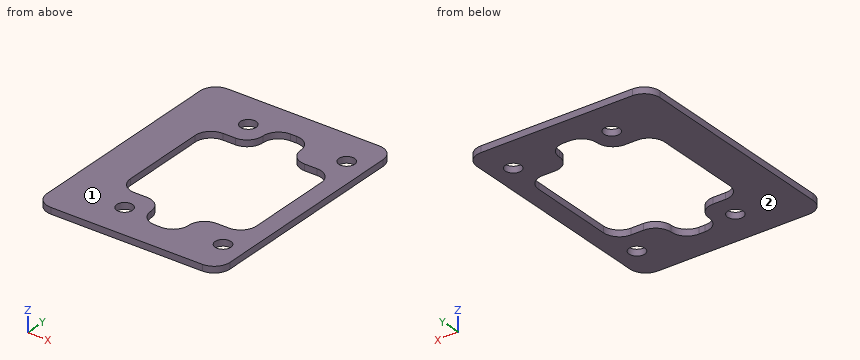
from build123d import *

# Parameters (mm, degrees)
SKETCH1_W       = 23.25
SKETCH1_H       = 30
SKETCH1_R       = 1
BODY_DEPTH      = 0.8
CORNER_FILLET_R = 2
CUTOUT_DEPTH    = 49.678263528
CUTOUT_FILLET_R = 2


with BuildPart() as part:
    # Sketch1 → body (new body)
    with BuildSketch(Plane.XY):
        with Locations((16.812358178, 24.5)):
            Rectangle(SKETCH1_W, SKETCH1_H)
        with Locations((25.687358178, 14)):
            Circle(SKETCH1_R, mode=Mode.SUBTRACT)
        with Locations(Location((25.687358178, 35, 0), (0, 0, 180))):
            Circle(SKETCH1_R, mode=Mode.SUBTRACT)
        with Locations(Location((13.187358178, 14, 0), (0, 0, 180))):
            Circle(SKETCH1_R, mode=Mode.SUBTRACT)
        with Locations((13.187358178, 35)):
            Circle(SKETCH1_R, mode=Mode.SUBTRACT)
    extrude(amount=BODY_DEPTH)

    # corner fillet
    corner_fillet_edges = [part.edges().sort_by_distance(p)[0] for p in [
        (5.187358178, 39.5, 0.4),
        (28.437358178, 39.5, 0.4),
        (28.437358178, 9.5, 0.4),
        (5.187358178, 9.5, 0.4),
    ]]
    fillet(corner_fillet_edges, radius=CORNER_FILLET_R)

    # Sketch2 → cutout (cut, through all)
    with BuildSketch(Plane(origin=(0, 0, 0), x_dir=(-1, 0, 0), z_dir=(0, 0, -1))):
        Polygon((-26.187358178, 17), (-26.187358178, 32), (-20.587358178, 32), (-20.587358178, 36), (-15.787358178, 36), (-15.787358178, 32), (-10.187358178, 32), (-10.187358178, 17), (-15.787358178, 17), (-15.787358178, 13), (-20.587358178, 13), (-20.587358178, 17), align=None)
    extrude(amount=-CUTOUT_DEPTH, mode=Mode.SUBTRACT)

    # cutout fillet
    cutout_fillet_edges = [part.edges().sort_by_distance(p)[0] for p in [
        (26.187358178, 32, 0.4),
        (20.587358178, 32, 0.4),
        (20.587358178, 36, 0.4),
        (15.787358178, 36, 0.4),
        (15.787358178, 32, 0.4),
        (10.187358178, 32, 0.4),
        (10.187358178, 17, 0.4),
        (15.787358178, 17, 0.4),
        (15.787358178, 13, 0.4),
        (20.587358178, 13, 0.4),
        (20.587358178, 17, 0.4),
        (26.187358178, 17, 0.4),
    ]]
    fillet(cutout_fillet_edges, radius=CUTOUT_FILLET_R - 0.0001)  # a hair under: the kernel refuses the full size


solid = part.part
Work out the finished part from the listing and answer in its coordinate system (mm). Face numbers are marked on the shaded views. Coordinates: 2 decimals unless noted, no trailing zeros. Loops run counter-clockwise (first coordinate to the right, second up) from the corner with the lowest first, then second, coordinate; pieces in that order, holes last. Notation, with made-up numbers: M -17,-9 L 23,-9 A26 ccw 23,28 Z; hole C 5.5,85 d7. An arc over 180 degrees is marked long. Answer in a Markdown table with one row per item. Add a question column.
1. Consider L1, parallel to X at y = 28.5, z = 0.1; L2, parallel to X at y = 14.5, z = 0.3; L3, parallel to Y at x = 17.75, z = 0.35. Determine where each line is inside the solid, lowest interval first.
2. Flat-ended cylindrical pins translate along their axes: P1, Ø2.5, axis at x = 13.19, y = 14, coming from the +Z side; P2, Ø1.8, axis at x = 13.19, y = 35, coming from the +Z side. Find the tip coordinate at first contact, or state that the pin passes through.
3. Find section D-D, the plane z = 0.2. State how many separate pieces and enclosed holes the cut face has, then the cut area to 3 significant figures.
4. Find section B-B, the plane y = 35. Write down the section's boundary in (x, z), then the cut area to 3 significant figures.
5. The mould has two halves that part along Z. Classify the marked faces 1 and 2: pulls with the +Z half, pulls with the -Z half, needs draft (parallel to the pull), parting line crosses it, or undercut.
6. Find section C-C, the plane x = 14.75. Write down the section's boundary in (y, z), then the cut area to 3 significant figures.
7. Find section A-A, the plane y = 21. Write down the section's boundary in (x, z).
Reported:
| question | item | result |
|---|---|---|
| 1 | L1 | x = 5.19 to 10.19, 26.19 to 28.44 |
| 1 | L2 | x = 5.19 to 12.32, 14.05 to 15.85, 20.52 to 24.82, 26.55 to 28.44 |
| 1 | L3 | y = 9.5 to 13, 36 to 39.5 |
| 2 | P1 | stops at z = 0.8 |
| 2 | P2 | passes through |
| 3 | separate pieces | 1 |
| 3 | enclosed holes | 5 |
| 3 | area | 407 mm^2 |
| 4 | outline | M 5.19,0 L 12.19,0 L 12.19,0.8 L 5.19,0.8 Z; M 14.19,0 L 16.06,0 L 16.06,0.8 L 14.19,0.8 Z; M 20.32,0 L 24.69,0 L 24.69,0.8 L 20.32,0.8 Z; M 26.69,0 L 28.44,0 L 28.44,0.8 L 26.69,0.8 Z |
| 4 | area | 12.0 mm^2 |
| 5 | face 1 | pulls with the +Z half |
| 5 | face 2 | pulls with the -Z half |
| 6 | outline | M 9.5,0 L 16.75,0 L 16.75,0.8 L 9.5,0.8 Z; M 32.25,0 L 39.5,0 L 39.5,0.8 L 32.25,0.8 Z |
| 6 | area | 11.6 mm^2 |
| 7 | outline | M 5.19,0 L 10.19,0 L 10.19,0.8 L 5.19,0.8 Z; M 26.19,0 L 28.44,0 L 28.44,0.8 L 26.19,0.8 Z |
